For this review, take the finished solid that the model builds, in its own axes (mm). Face numbers are marked on the shaded views. A direction names the side the tool comes from. Give positions to 0.01 mm unless a question says otherwise; leave off trailing zeros. Order: outer loops, then holes, each group sorted by start corner. A loop starts at its lowest first (then second) coordinate and runs counter-clockwise, first axis right, second up. Notation, with made-up numbers: M -15.5,45.25 L -11.5,45.25 A30 ccw -11.5,75.25 Z; hole C 82.5,29 d6. An arc over 180 degrees is marked long. Answer as CSV lines item,"result". Start each with the question number.
1. We need section C-C, the plane y = 0.5. Give the boundary of the cut face in (x, z), and give its area (3 significant figures).
2. We need section B-B, the plane z = 1.25. Give the boundary of the cut face in (x, y).
3. Clearance check with flat-ended pins moving along their axes: P1, Ø1, axis at x = -1.5, y = 0.5, coming from the +Z side; P2, Ø6, axis at x = 0, z = -4.5, coming from the -Y side; P3, Ø8, axis at x = -5.5, z = -9.5, coming from the +Y side; P4, Ø2, axis at y = -3, z = -3, coming from the -X side. State where each tip first meets the part, or that it passes through.
4. Machinability: for the marked faces 1 and 2, which of the approach directions +Z, -Z, +X, -X, +Y, -Y give a long, thin tool a straight path to every point of the face, cutting with its end or side? Answer none if there is none.
5. We need section A-A, the plane x = 0. Give the boundary of the cut face in (y, z).
6. Mouldability with a two-part tool opening along X and no side actions: class the marked faces 3, 4, 5 and 6 as pulls with the +X half, pulls with the -X half, needs draft (parallel to the pull), parting line crosses it, or undercut.
7. For line 1 along Z through (x, y) = (0, -3.65); line 2 along Y through (x, z) = (-1.75, -9); line 3 along Y through (x, z) = (2, -0.75), list the stretches that pass through material, from the lowest coordinate up.
8. We need section D-D, the plane y = -2.75. Give the boundary of the cut face in (x, z).
from build123d import *

# Parameters (mm, degrees)
BOSS_EXTRUDE1_DEPTH = 6
SKETCH2_R           = 5
BOSS_EXTRUDE2_DEPTH = 12
SKETCH3_R           = 2.5
CUT_EXTRUDE1_DEPTH  = 12
SKETCH4_R           = 1.65
CUT_EXTRUDE2_DEPTH  = 6
SKETCH5_R           = 1.25
CUT_EXTRUDE3_DEPTH  = 5.1


with BuildPart() as part:
    # Sketch1 → Boss-Extrude1 (new body)
    with BuildSketch(Plane.XY):
        Polygon((6.92820323, 0), (3.464101615, 6), (-3.464101615, 6), (-6.92820323, 0), (-3.464101615, -6), (3.464101615, -6), align=None)
    extrude(amount=BOSS_EXTRUDE1_DEPTH)

    # Sketch2 → Boss-Extrude2 (add)
    with BuildSketch(Plane.XY):
        Circle(SKETCH2_R)
    extrude(amount=-BOSS_EXTRUDE2_DEPTH)

    # Sketch3 → Cut-Extrude1 (cut)
    with BuildSketch(Plane.XY):
        Circle(SKETCH3_R)
    extrude(amount=-CUT_EXTRUDE1_DEPTH, mode=Mode.SUBTRACT)

    # Sketch4 → Cut-Extrude2 (cut)
    with BuildSketch(Plane.XY):
        Circle(SKETCH4_R)
    extrude(amount=CUT_EXTRUDE2_DEPTH, mode=Mode.SUBTRACT)

    # Sketch5 → Cut-Extrude3 (cut)
    with BuildSketch(Plane(origin=(0, 0, 0), x_dir=(1, 0, 0), z_dir=(0, 1, 0))):
        with Locations(Location((0, 9, 0), (0, 0, 270))):
            Circle(SKETCH5_R)
    extrude(amount=-CUT_EXTRUDE3_DEPTH, mode=Mode.SUBTRACT)


solid = part.part
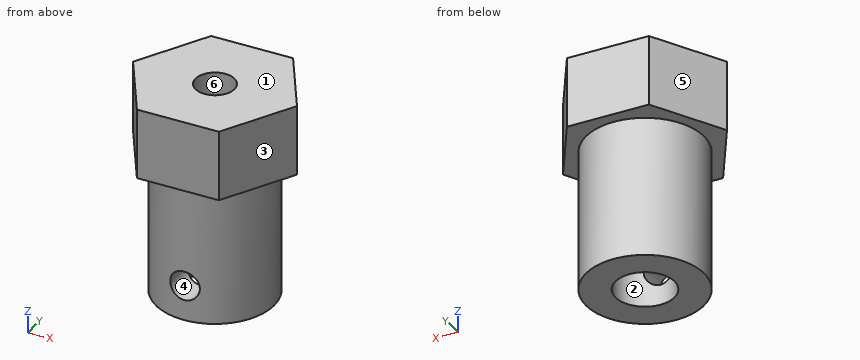
Result set:
1,outline,"M -6.64,0 L -4.97,0 L -4.97,-12 L -2.45,-12 L -2.45,0 L -1.57,0 L -1.57,6 L -6.64,6 Z; M 1.57,0 L 2.45,0 L 2.45,-12 L 4.97,-12 L 4.97,0 L 6.64,0 L 6.64,6 L 1.57,6 Z"
1,area,"121 mm2"
2,outline,"M -6.93,0 L -3.46,-6 L 3.46,-6 L 6.93,0 L 3.46,6 L -3.46,6 Z; hole C 0,0 d3.3"
3,P1,"z = 6"
3,P2,"y = -5"
3,P3,"y = 4.77"
3,P4,"x = -4.58"
4,face 1,"+Z, +X, -X, +Y, -Y"
4,face 2,"-Z"
5,outline,"M -6,0 L -5,0 L -5,-7.75 L -2.5,-7.75 L -2.5,0 L -1.65,0 L -1.65,6 L -6,6 Z; M -5,-12 L -2.5,-12 L -2.5,-10.25 L -5,-10.25 Z; M 1.65,0 L 2.5,0 L 2.5,-12 L 5,-12 L 5,0 L 6,0 L 6,6 L 1.65,6 Z"
6,face 3,"pulls with the +X half"
6,face 4,"undercut"
6,face 5,"pulls with the -X half"
6,face 6,"undercut"
7,line 1,"-12 to -10.25, -7.75 to 6"
7,line 2,"-4.68 to -1.79, 1.79 to 4.68"
7,line 3,"-4.58 to -1.5, 1.5 to 4.58"
8,outline,"M -5.34,0 L -4.18,0 L -4.18,-12 L 4.18,-12 L 4.18,0 L 5.34,0 L 5.34,6 L -5.34,6 Z; hole C 0,-9 d2.5"
